For this review, take the finished solid that the model builds, in its own axes (mm). A direction names the side the tool comes from. Round coordinates to 2 decimals unless told otherwise and drop trailing zeros. Loops run counter-clockwise (first coordinate to the right, second up) from the corner with the lowest first, then second, coordinate; pieces in that order, holes last. Notation, with made-up numbers: M 60.5,84.5 L 70.5,84.5 A16 ccw 70.5,88.5 Z; hole C 21,66 d6. An arc over 180 degrees is marked long. One line per question, with ' | ' between items. Start each with the question number.
1) For faces 5 (the face through (5, 129, -69)), 6 (the face through (1.188, 1.644, -69.02)), list the 3-axis set-ups (+Z, -Z, +X, -X, +Y, -Y) from which the entire face can be reached by the end or side of a thin tool; tool diameter is ignored.
2) For probe 1 along Z at (x, y) = (-15, 85.5); probe 2 along Y at (x, z) = (-1, -36.5); probe 3 along Y at (x, z) = (-32.5, -9), list the stretches that pass through material, from the lowest coordinate up. Write a range as from..to.
3) For pin 1 Ø5 at (x, z) = (-15.5, -118.5) entering from -Y; pin 2 Ø6 at (y, z) = (60.5, -110.5) entering from +X; pin 3 Ø12 at (y, z) = (134, -43) entering from +X, all flat-tipped, find the tip position at first contact; note any pin that passes through.
4) We need section C-C (z = -16). Give the boundary of the cut face in (x, y), and give its area (3 significant figures).
5) We need section A-A (z = -97). Give the boundary of the cut face in (x, y).
6) We need section D-D (y = 106). Give the boundary of the cut face in (x, z).
7) Mouldability with a two-part tool opening along Z and no side actions: class faces 1 (the face through (-20.192, 14.139, -69.02)), 2 (the face through (-22, 70, 0)), 3 (the face through (-15, 92, -108.5)), 4 (the face through (-24.676, 66.61, -66.614)) as pulls with the +Z half, pulls with the -Z half, needs draft (parallel to the pull), parting line crosses it, or undercut.
8) We need section B-B (x = -28.5). Give the boundary of the cut face in (y, z).
```python
from build123d import *

# Parameters (mm, degrees)
RESSALTO_EXTRUS_O1_DEPTH = 140
ESBO_O3_W                = 86
ESBO_O3_H                = 57
ESBO_O3_W_2              = 77
ESBO_O3_H_2              = 51
CORTE_EXTRUS_O1_DEPTH    = 2.5
ESBO_O4_W                = 77
ESBO_O4_H                = 51
CORTE_EXTRUS_O2_DEPTH    = 201.480317617
CORTE_EXTRUS_O3_DEPTH    = 210.721949933


with BuildPart() as part:
    # Esboço1 → Ressalto-extrusão1 (new body)
    with BuildSketch(Plane.XY):
        with BuildLine():
            Line((-41.646443714, 31.110299699), (9.909852794, 150.449933896))
            Line((9.909852794, 150.449933896), (13.581841538, 148.863586311))
            Line((13.581841538, 148.863586311), (-36.681468487, 32.516884972))
            ThreePointArc((-36.681468487, 32.516884972), (-36.769743597, 31.178562616), (-35.992626987, 30.085407091))
            Line((-35.992626987, 30.085407091), (2.342768013, 3.242674532))
            Line((2.342768013, 3.242674532), (0, 0))
            Line((0, 0), (-40.957602214, 28.678821818))
            ThreePointArc((-40.957602214, 28.678821818), (-41.734718825, 29.771977342), (-41.646443714, 31.110299699))
        make_face()
    extrude(amount=-RESSALTO_EXTRUS_O1_DEPTH)

    # Esboço3 → Corte-extrusão1 (cut)
    with BuildSketch(Plane(origin=(-42.750445362, 18.468756434, 0), x_dir=(0, 0, -1), z_dir=(0.9179971861354039, -0.39658689621252097, 0))):
        with Locations((70, 78.672876452)):
            Rectangle(ESBO_O3_W, ESBO_O3_H)
        with Locations((70, 78.672876452)):
            Rectangle(ESBO_O3_W_2, ESBO_O3_H_2, mode=Mode.SUBTRACT)
    extrude(amount=-CORTE_EXTRUS_O1_DEPTH, mode=Mode.SUBTRACT)

    # Esboço4 → Corte-extrusão2 (cut, through all)
    with BuildSketch(Plane(origin=(-42.750445362, 18.468756434, 0), x_dir=(0, 0, -1), z_dir=(0.9179971861354039, -0.39658689621252097, 0))):
        with Locations((70, 78.672876452)):
            Rectangle(ESBO_O4_W, ESBO_O4_H)
    extrude(amount=-CORTE_EXTRUS_O2_DEPTH, mode=Mode.SUBTRACT)

    # Esboço5 → Corte-extrusão3 (cut, through all)
    with BuildSketch(Plane.XY):
        Polygon((9.909852794, 150.449933896), (13.004458236, 147.527091708), (13.581841538, 148.863586311), align=None)
    extrude(amount=-CORTE_EXTRUS_O3_DEPTH, mode=Mode.SUBTRACT)


solid = part.part
```
Answers below:
1) face 5: +Z, -Z, +X | face 6: +Z, -Z, +X, -Y
2) probe 1: -140..-113, -27..0 | probe 2: 0.7..5.58, 117.18..125.2 | probe 3: 22.76..27.64, 42.2..52.28
3) pin 1: y = 9.1 | pin 2: x = -23.3 | pin 3: x = 9.75
4) outline: M -41.65,31.11 A2 ccw -40.96,28.68 L 0,0 L 2.34,3.24 L -35.99,30.09 A2 cw -36.68,32.52 L 13,147.53 L 9.91,150.45 Z | area: 717 mm^2
5) outline: M -41.65,31.11 A2 ccw -40.96,28.68 L 0,0 L 2.34,3.24 L -35.99,30.09 A2 cw -36.68,32.52 L -22.85,64.53 L -25.15,65.52 L -23.96,68.27 L -25.33,68.87 Z; M -5.11,115.69 L -3.73,115.09 L -2.54,117.84 L -0.25,116.85 L 13,147.53 L 9.91,150.45 Z
6) outline: M -9.29,-140 L -4.94,-140 L -4.94,-113 L -7.66,-113 L -7.66,-108.5 L -9.29,-108.5 Z; M -9.29,-31.5 L -7.66,-31.5 L -7.66,-27 L -4.94,-27 L -4.94,0 L -9.29,0 Z
7) face 1: needs draft | face 2: pulls with the +Z half | face 3: undercut | face 4: undercut
8) outline: M 19.96,-140 L 24.84,-140 L 24.84,0 L 19.96,0 Z; M 51.45,-140 L 61.54,-140 L 61.54,0 L 51.45,0 Z
